Verification items for this drawing (mm, ordinates from the low corner). Coordinates: 2 decimals unless noted, no trailing zeros. Write each loop counter-clockwise with the first axis right and the second up, starting at its lowest first coordinate (ties: lowest second). Pieces come first, ordered by that corner, then holes. Notation, with made-up numbers: M -4,-35.5 L 7,-35.5 A32 ccw 7,-1.5 Z; hole C 84.5,-38.5 d9. An arc over 180 degrees is marked long. Answer as CSV lines item,"result". Start each with the question number.
1) Section check B-B (y = 6). Record the cut outline in (x, z).
2) Section check C-C (x = 3). Record the cut outline in (y, z), and give its area (3 significant figures).
3) Section check A-A (z = 25.5). Record the cut outline in (x, y), and give its area (3 significant figures).
4) Material ranges on L1, parallel to X at y = 4.25, z = 14; L2, parallel to X at y = 2.25, z = 23; L3, parallel to Y at x = 1, z = 30.5, recorded low to high. Write a range as [from, to].
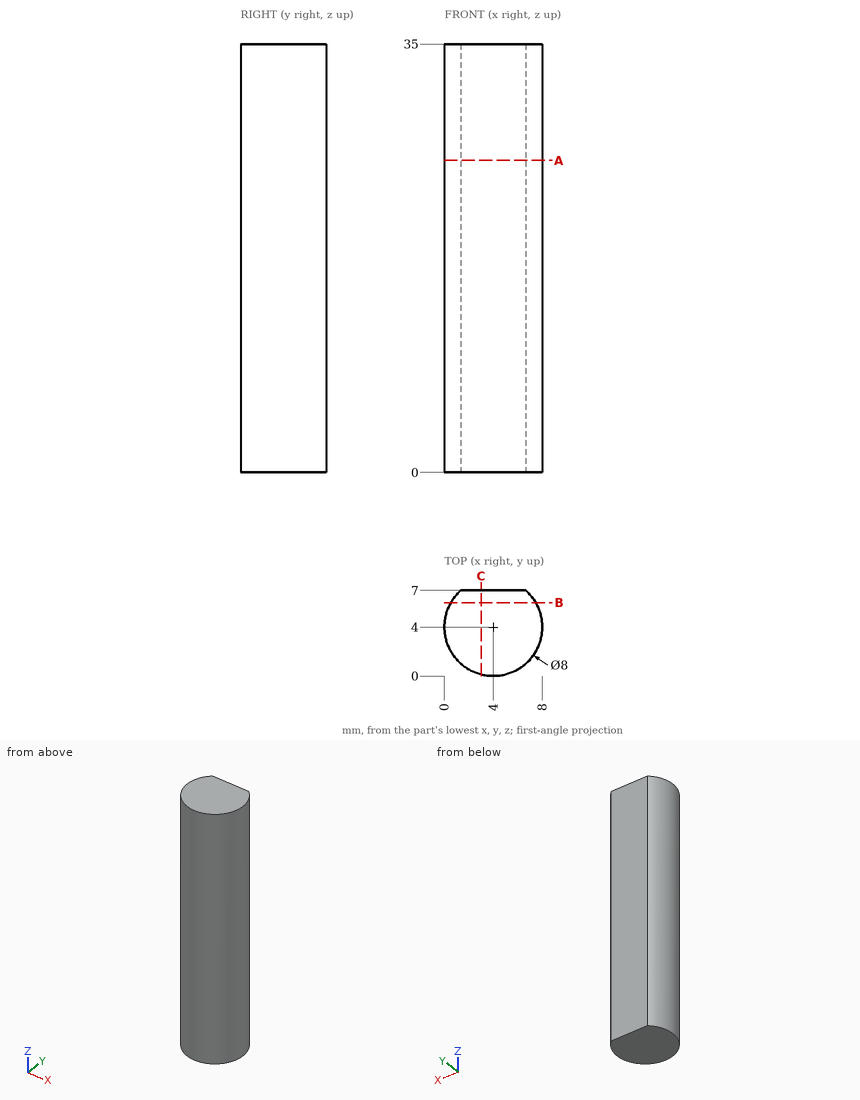
Results found:
1,outline,"M 0.54,0 L 7.46,0 L 7.46,35 L 0.54,35 Z"
2,outline,"M 0.13,0 L 7,0 L 7,35 L 0.13,35 Z"
2,area,"241 mm2"
3,outline,"M 1.35,7 A4 ccw long 6.65,7 Z"
3,area,"46.6 mm2"
4,L1,"x = [0.01, 7.99]"
4,L2,"x = [0.4, 7.6]"
4,L3,"y = [1.35, 6.65]"
